```python
from build123d import *

# Parameters (mm, degrees)
F0_W     = 18
F0_H     = 40
F1_DEPTH = 5
F2_R     = 1.75
F3_DEPTH = 5
F4_W     = 18
F4_H     = 10
F5_DEPTH = 20
F6_R     = 5.75
F7_DEPTH = 10
F8_SIZE  = 0.5


with BuildPart() as f1:
    # F0 (on Front) → F1 (new body)
    with BuildSketch(Plane.XZ):
        Rectangle(F0_W, F0_H)
    extrude(amount=F1_DEPTH)

    # F2 (on face) → F3 (cut, through all)
    with BuildSketch(Plane.XZ.offset(5)):
        with Locations((-4, -15)):
            Circle(F2_R)
        with Locations((4, -15)):
            Circle(F2_R)
        with Locations((4, -7)):
            Circle(F2_R)
        with Locations((-4, -7)):
            Circle(F2_R)
    extrude(amount=-F3_DEPTH, mode=Mode.SUBTRACT)

    # F4 (on face) → F5 (join)
    with BuildSketch(Plane.XZ.offset(5)):
        with Locations((0, 15)):
            Rectangle(F4_W, F4_H)
    extrude(amount=F5_DEPTH)

    # F6 (on face) → F7 (cut, through all)
    with BuildSketch(Plane(origin=(0, 0, 10), x_dir=(1, 0, 0), z_dir=(0, 0, -1))):
        with Locations((0, 16)):
            Circle(F6_R)
    extrude(amount=-F7_DEPTH, mode=Mode.SUBTRACT)

    # F8
    f8_edges = [f1.edges().sort_by_distance(p)[0] for p in [
        (9, -15, 10),
        (-9, -15, 10),
        (0, -25, 10),
        (9, -25, 15),
        (-9, -25, 15),
        (0, -25, 20),
        (9, -12.5, 20),
        (9, -5, -5),
        (9, 0, 0),
        (0, 0, -20),
        (9, -2.5, -20),
        (0, -5, -20),
        (-9, -2.5, -20),
        (-9, -5, -5),
        (-9, 0, 0),
        (-9, -12.5, 20),
        (0, 0, 20),
        (0, -5, 10),
        (-5.75, -16, 10),
    ]]
    chamfer(f8_edges, length=F8_SIZE)


solid = f1.part
```
The listing builds one solid part. Answer for the finished solid, in the listing's coordinates (mm). A direction names the side the tool comes from. Coordinates: 2 decimals unless noted, no trailing zeros. Write each loop counter-clockwise with the first axis right and the second up, starting at its lowest first coordinate (ties: lowest second). Pieces come first, ordered by that corner, then holes. Notation, with made-up numbers: (5, 53.25) - (47, 53.25) arc R34 cw to (47, 85.25) - close; hole circle Ø2 at (-1, 81.5). An arc over 180 degrees is marked (long way). Return JSON: item names as keys, results as strings. Group by question number.
1. Straight lines are drawn through the part: L1, parallel to Z at x = 4, y = -3.1; L2, parallel to Y at x = 0, z = 16; L3, parallel to Z at x = 5.25, y = -2. For each, find the intervals that lie inside material, in ascending order.
2. A cutting plane is placed at C-C, the plane y = -16. Determine the outline of the cut face in (x, z), plus the area to 4 significant figures.
3. A cutting plane is placed at B-B, the plane x = 0. Determine the outline of the cut face in (y, z).
4. A cutting plane is placed at D-D, the plane x = -7.5. Determine the outline of the cut face in (y, z), plus the area to 4 significant figures.
5. Which of the six approach directions +Z, -Z, +X, -X, +Y, -Y give full straight-line access (tool end or side, diameter ignored) to faces 1 (the flat face through (-9, -4, 8)), 2 (the flat face through (0, -5, -5))?
6. Determine the mould class of faces 3 (the cylindrical face through (3.772, -2.535, -13.265)), 4 (the flat face through (0, -10, 20)), 5 (the flat face through (4, -11, 10)) for opening direction Z: released by +Z, released by -Z, zero draft, split by the parting line, or undercut.
7. A cutting plane is placed at A-A, the plane z = -15. Determine the outline of the cut face in (x, y), plus the area to 3 significant figures.
8. Given pin 1 (4 mm diameter, centred on y = -8.5, z = 0, fed in from -X); pin 2 (4 mm diameter, centred on x = -5, y = -22.5, fed in from -Z); pin 3 (8.5 mm diameter, centred on x = 1, z = 1.5, fed in from -Y); pin 4 (1.5 mm diameter, centred on x = -4, y = -12.5, fed in from -Z), each flat-ended and moving along its own axis, determine where each tip first touches the part or whether it passes through.
Ans:
{
 "1": {"L1": "-20 to -16.75, -13.25 to -8.75, -5.25 to 20", "L2": "-25 to -21.75, -10.25 to 0", "L3": "-20 to -16.22, -13.78 to -8.22, -5.78 to 20"},
 "2": {"outline": "(-9, 10.5) - (-8.5, 10) - (-6.25, 10) - (-5.75, 10.5) - (-5.75, 20) - (-8.5, 20) - (-9, 19.5) - close; (5.75, 10.5) - (6.25, 10) - (8.5, 10) - (9, 10.5) - (9, 19.5) - (8.5, 20) - (5.75, 20) - close", "area": "64.25 mm²"},
 "3": {"outline": "(-25, 10.5) - (-24.5, 10) - (-22.25, 10) - (-21.75, 10.5) - (-21.75, 20) - (-24.5, 20) - (-25, 19.5) - close; (-10.25, 10.5) - (-9.75, 10) - (-5.5, 10) - (-5, 9.5) - (-5, -19.5) - (-4.5, -20) - (-0.5, -20) - (0, -19.5) - (0, 19.5) - (-0.5, 20) - (-10.25, 20) - close"},
 "4": {"outline": "(-25, 10.5) - (-24.5, 10) - (-5.5, 10) - (-5, 9.5) - (-5, -19.5) - (-4.5, -20) - (-0.5, -20) - (0, -19.5) - (0, 19.5) - (-0.5, 20) - (-24.5, 20) - (-25, 19.5) - close", "area": "399.5 mm²"},
 "5": {"face 1": "+Z, -Z, -X, +Y, -Y", "face 2": "-Z, +X, -X, -Y"},
 "6": {"face 3": "undercut", "face 4": "released by +Z", "face 5": "released by -Z"},
 "7": {"outline": "(-9, -4.5) - (-8.5, -5) - (-5.75, -5) - (-5.75, 0) - (-8.5, 0) - (-9, -0.5) - close; (-2.25, -5) - (2.25, -5) - (2.25, 0) - (-2.25, 0) - close; (5.75, -5) - (8.5, -5) - (9, -4.5) - (9, -0.5) - (8.5, 0) - (5.75, 0) - close", "area": "54.5 mm²"},
 "8": {"pin 1": "through", "pin 2": "z = 10", "pin 3": "y = -5", "pin 4": "z = 10.18"}
}
